from build123d import *

# Parameters (mm, degrees)
BOSS_EXTRUDE1_DEPTH      = 31.75
CUT_EXTRUDE2_DEPTH       = 115.012526534
CUT_EXTRUDE2_DEPTH_BACK  = 115.012526534
SKETCH4_R                = 6.35
CUT_EXTRUDE3_DEPTH       = 88.332955112
CUT_EXTRUDE13_DEPTH      = 31.75
CUT_EXTRUDE18_DEPTH      = 25.4
CUT_EXTRUDE22_DEPTH      = 88.332955112
CUT_EXTRUDE22_DEPTH_BACK = 25.4
CUT_EXTRUDE23_DEPTH      = 25.4
SKETCH14_R               = 4.7625
CUT_EXTRUDE24_DEPTH      = 114.470708815
SKETCH15_R               = 4.7625
CUT_EXTRUDE25_DEPTH      = 114.470708815


with BuildPart() as part:
    # Sketch2 → Boss-Extrude1 (new body)
    with BuildSketch(Plane.XY):
        Polygon((-77.635875696, 41.712828345), (-64.935875696, 41.712828345), (-64.935875696, 6.683574613), (-39.535875696, 6.683574613), (-39.535875696, 41.10626118), (-26.835875696, 41.10626118), (-26.835875696, -9.69373882), (-7.785875696, -9.69373882), (-7.785875696, -22.39373882), (-36.360875696, -22.39373882), (-36.360875696, -6.016425387), (-68.110875696, -6.016425387), (-68.110875696, -21.787171655), (-96.685875696, -21.787171655), (-96.685875696, -9.087171655), (-77.635875696, -9.087171655), align=None)
    extrude(amount=BOSS_EXTRUDE1_DEPTH)

    # Sketch3 → Cut-Extrude2 (cut, two sides: drawn at the far end of the back side and taken through both)
    with BuildSketch(Plane(origin=(0, -9.69373882, 0), x_dir=(1, 0, 0), z_dir=(0, 1, 0)).offset(-CUT_EXTRUDE2_DEPTH_BACK)):
        Polygon((-96.685875696, -24.13), (-89.065875696, -31.75), (-96.685875696, -31.75), align=None)
        Polygon((-15.405875696, -31.75), (-7.785875696, -31.75), (-7.785875696, -24.13), align=None)
    extrude(amount=CUT_EXTRUDE2_DEPTH + CUT_EXTRUDE2_DEPTH_BACK, mode=Mode.SUBTRACT)

    # Sketch4 → Cut-Extrude3 (cut, through all)
    with BuildSketch(Plane(origin=(-26.835875696, 0, 0), x_dir=(0, 0, -1), z_dir=(1, 0, 0))):
        with Locations(Location((-15.875, 28.40626118, 0), (0, 0, 90))):
            Circle(SKETCH4_R)
    extrude(amount=-CUT_EXTRUDE3_DEPTH, mode=Mode.SUBTRACT)

    # Sketch9 → Cut-Extrude13 (cut)
    with BuildSketch(Plane(origin=(-26.835875696, 0, 0), x_dir=(0, 0, -1), z_dir=(1, 0, 0))):
        with BuildLine():
            Line((-31.75, 41.10626118), (-31.75, 32.743943383))
            ThreePointArc((-31.75, 32.743943383), (-24.905282657, 38.886336135), (-15.980537449, 41.10626118))
            Line((-15.980537449, 41.10626118), (-31.75, 41.10626118))
        make_face()
    extrude(amount=-CUT_EXTRUDE13_DEPTH, mode=Mode.SUBTRACT)

    # Sketch10 → Cut-Extrude18 (cut)
    with BuildSketch(Plane(origin=(-26.835875696, 0, 0), x_dir=(0, 0, -1), z_dir=(1, 0, 0))):
        with BuildLine():
            Line((0, 32.58654489), (0, 41.10626118))
            Line((0, 41.10626118), (-15.980537449, 41.10626118))
            ThreePointArc((-15.980537449, 41.10626118), (-6.9256611, 38.843300754), (0, 32.58654489))
        make_face()
    extrude(amount=-CUT_EXTRUDE18_DEPTH, mode=Mode.SUBTRACT)

    # Sketch11 → Cut-Extrude22 (cut, two sides: drawn at the far end of the back side and taken through both)
    with BuildSketch(Plane.ZY.offset(77.635875696).offset(-CUT_EXTRUDE22_DEPTH_BACK)):
        Polygon((-151.990316571, 41.10626118), (0, 41.10626118), (31.75, 41.10626118), (183.740316571, 41.10626118), (183.740316571, 345.086894323), (-151.990316571, 345.086894323), align=None)
    extrude(amount=CUT_EXTRUDE22_DEPTH + CUT_EXTRUDE22_DEPTH_BACK, mode=Mode.SUBTRACT)

    # Sketch13 → Cut-Extrude23 (cut)
    with BuildSketch(Plane.ZY.offset(77.635875696)):
        with BuildLine():
            Line((31.75, 41.10626118), (15.875, 41.10626118))
            ThreePointArc((15.875, 41.10626118), (24.883346001, 38.841737114), (31.75, 32.58654489))
            Line((31.75, 32.58654489), (31.75, 41.10626118))
        make_face()
        with BuildLine():
            Line((15.875, 41.10626118), (0, 41.10626118))
            Line((0, 41.10626118), (0, 32.58654489))
            ThreePointArc((0, 32.58654489), (6.866653999, 38.841737114), (15.875, 41.10626118))
        make_face()
    extrude(amount=-CUT_EXTRUDE23_DEPTH, mode=Mode.SUBTRACT)

    # Sketch14 → Cut-Extrude24 (cut, through all)
    with BuildSketch(Plane(origin=(0, -9.087171655, 0), x_dir=(1, 0, 0), z_dir=(0, 1, 0))):
        with Locations(Location((-17.310875696, -15.875, 0), (0, 0, 180))):
            Circle(SKETCH14_R)
    extrude(amount=-CUT_EXTRUDE24_DEPTH, mode=Mode.SUBTRACT)

    # Sketch15 → Cut-Extrude25 (cut, through all)
    with BuildSketch(Plane(origin=(0, -9.087171655, 0), x_dir=(1, 0, 0), z_dir=(0, 1, 0))):
        with Locations(Location((-87.160875696, -15.875, 0), (0, 0, 180))):
            Circle(SKETCH15_R)
    extrude(amount=-CUT_EXTRUDE25_DEPTH, mode=Mode.SUBTRACT)


solid = part.part
For this review, take the finished solid that the model builds, in its own axes (mm). A direction names the side the tool comes from. Give positions to 0.01 mm unless a question says otherwise; leave off trailing zeros. Order: outer loops, then holes, each group sorted by start corner. A loop starts at its lowest first (then second) coordinate and runs counter-clockwise, first axis right, second up. Notation, with made-up numbers: M 15.5,40 L 69.5,40 A23 ccw 69.5,75 Z; hole C -12.75,35 d6. An arc over 180 degrees is marked long. Answer in a Markdown table with one row per item. Add a question column.
(1) For pin 1 (11 mm diameter, centred on x = -87.16, z = 15.88, fed in from +Y); pin 2 (7.5 mm diameter, centred on x = -17.31, z = 15.88, fed in from +Y); pin 3 (1 mm diameter, centred on y = -5, z = 17.5, fed in from +X); pin 4 (10 mm diameter, centred on x = -35.5, z = 8, fed in from +Y), all flat-tipped, find the tip position at first contact; note any pin that passes through.
(2) Consider section A-A on y = -15. Give the number of separate pieces and of enclosed holes in the cut face, and give its area (3 significant figures).
(3) Mouldability with a two-part tool opening along Y and no side actions: class faces 1 (the face through (-11.543, -16.133, 27.887)), 2 (the face through (-52, -6.016, 16)), 3 (the face through (-71.2, 34.27, 13.44)), 4 (the face through (-52, 6.684, 16)) as +Y half, -Y half, draft (parallel to the pull), parting line (faces both ways), or undercut.
(4) Consider section B-B on y = 9.5. State the section outline as (x, z) points, and give its area (3 significant figures).
(5) Consider section D-D on y = 24.5. State the section outline as (x, z) points.
(6) For faces 5 (the face through (-22, -9.694, 12)), 6 (the face through (-64.936, 20, 16)), 7 (the face through (-77.636, 16, 16)), 8 (the face through (-68.111, -14, 16)), list the 3-axis set-ups (+Z, -Z, +X, -X, +Y, -Y) from which the entire face can be reached by the end or side of a thin tool; tool diameter is ignored.
(7) Consider section C-C on x = -20.5. State the section outline as (y, z) points, and give its area (3 significant figures).
(8) Wall thickness on probe 1 along X at (y, z) = (-9, 21.5); probe 2 along X at (y, z) = (27, 3); probe 3 along X at (y, z) = (-20, 18.5): over which ranges is each line inside the solid? List them lowest first. Write a range as [from, to].
Evaluation:
| question | item | result |
|---|---|---|
| 1 | pin 1 | stops at y = -9.09 |
| 1 | pin 2 | passes through |
| 1 | pin 3 | stops at x = -26.84 |
| 1 | pin 4 | stops at y = 40.87 |
| 2 | separate pieces | 2 |
| 2 | enclosed holes | 2 |
| 2 | area | 1,610 mm^2 |
| 3 | face 1 | draft |
| 3 | face 2 | -Y half |
| 3 | face 3 | undercut |
| 3 | face 4 | +Y half |
| 4 | outline | M -77.64,0 L -64.94,0 L -64.94,31.75 L -77.64,31.75 Z; M -39.54,0 L -26.84,0 L -26.84,31.75 L -39.54,31.75 Z |
| 4 | area | 806 mm^2 |
| 5 | outline | M -77.64,0 L -64.94,0 L -64.94,10.87 L -77.64,10.87 Z; M -77.64,20.88 L -64.94,20.88 L -64.94,31.75 L -77.64,31.75 Z; M -39.54,0 L -26.84,0 L -26.84,10.87 L -39.54,10.87 Z; M -39.54,20.88 L -26.84,20.88 L -26.84,31.75 L -39.54,31.75 Z |
| 6 | face 5 | +Z, -Z, +X, +Y |
| 6 | face 6 | +Z, -Z, +Y |
| 6 | face 7 | +Z, -Z, -X, +Y |
| 6 | face 8 | +Z, -Z, -Y |
| 7 | outline | M -22.39,0 L -9.69,0 L -9.69,12.34 L -22.39,12.34 Z; M -22.39,19.41 L -9.69,19.41 L -9.69,31.75 L -22.39,31.75 Z |
| 7 | area | 313 mm^2 |
| 8 | probe 1 | x = [-77.64, -68.11], [-36.36, -26.84] |
| 8 | probe 2 | x = [-77.64, -64.94], [-39.54, -26.84] |
| 8 | probe 3 | x = [-96.69, -91.13], [-83.19, -68.11], [-36.36, -21.28], [-13.34, -7.79] |
